Geometry: final body of the model. Coordinates: model frame, mm. Face numbers are marked on the shaded views. A direction names the side the tool comes from. Give positions to 0.01 mm unless a question says otherwise; leave off trailing zeros. Write each loop counter-clockwise with the first axis right and the second up, starting at its lowest first coordinate (ties: lowest second). Pieces come first, ordered by that corner, then holes. Notation, with made-up numbers: M 22.25,-15.75 L 67.25,-15.75 A26 cw 67.25,11.25 Z; hole C 76.25,86 d4. An arc over 180 degrees is marked long. Answer as a JSON object with one key per item and string values.
from build123d import *

# Parameters (mm, degrees)
BASE_FLANGE1_DEPTH = 12.319
FILLET1_RADIUS     = 12.319
FILLET1_LENGTH     = 1.524
FILLET2_RADIUS     = 12.319
FILLET2_LENGTH     = 1.524
SKETCH3_R          = 4.0132
SKETCH3_R_2        = 1.143
EXTRUDE1_DEPTH     = 68.388191377
SKETCH4_R          = 4.0132
SKETCH4_R_2        = 1.143
EXTRUDE2_DEPTH     = 1.524


# Sheet-metal steps are written as plain solids
with BuildPart() as part:
    # Sketch1 → Base-Flange1 (new, symmetric)
    with BuildSketch(Plane.XY):
        with BuildLine():
            Line((-26.162, 40.64), (-26.162, 2.3368))
            ThreePointArc((-26.162, 2.3368), (-25.477567126, 0.684432874), (-23.8252, 0))
            Line((-23.8252, 0), (23.8252, 0))
            ThreePointArc((23.8252, 0), (25.477567126, 0.684432874), (26.162, 2.3368))
            Line((26.162, 2.3368), (26.162, 40.64))
            Line((26.162, 40.64), (24.638, 40.64))
            Line((24.638, 40.64), (24.638, 2.3368))
            ThreePointArc((24.638, 2.3368), (24.399936392, 1.762063608), (23.8252, 1.524))
            Line((23.8252, 1.524), (-23.8252, 1.524))
            ThreePointArc((-23.8252, 1.524), (-24.399936392, 1.762063608), (-24.638, 2.3368))
            Line((-24.638, 2.3368), (-24.638, 40.64))
            Line((-24.638, 40.64), (-26.162, 40.64))
        make_face()
    extrude(amount=BASE_FLANGE1_DEPTH, both=True)

    # Fillet1: full round fillet: the end face becomes a half cylinder, R = half its width
    fillet1_face = Plane((-25.4, 40.64, 0), x_dir=(-1, 0, 0), z_dir=(0, 1, 0))  # on the end face: x along it, z out of the body
    fillet1_slab = fillet1_face.offset(-FILLET1_RADIUS / 2) * Box(FILLET1_LENGTH, 2 * FILLET1_RADIUS, FILLET1_RADIUS, mode=Mode.PRIVATE)  # the body's end, R deep
    fillet1_round = Plane((-25.4, 28.321, 0), x_dir=(0, 1, 0), z_dir=(-1, 0, 0)) * Cylinder(FILLET1_RADIUS, FILLET1_LENGTH, mode=Mode.PRIVATE)  # its axis R under the face
    add(fillet1_slab - fillet1_round, mode=Mode.SUBTRACT)

    # Fillet2: full round fillet: the end face becomes a half cylinder, R = half its width
    fillet2_face = Plane((25.4, 40.64, 0), x_dir=(-1, 0, 0), z_dir=(0, 1, 0))  # on the end face: x along it, z out of the body
    fillet2_slab = fillet2_face.offset(-FILLET2_RADIUS / 2) * Box(FILLET2_LENGTH, 2 * FILLET2_RADIUS, FILLET2_RADIUS, mode=Mode.PRIVATE)  # the body's end, R deep
    fillet2_round = Plane((25.4, 28.321, 0), x_dir=(0, 1, 0), z_dir=(-1, 0, 0)) * Cylinder(FILLET2_RADIUS, FILLET2_LENGTH, mode=Mode.PRIVATE)  # its axis R under the face
    add(fillet2_slab - fillet2_round, mode=Mode.SUBTRACT)

    # Sketch3 → Extrude1 (cut, through all)
    with BuildSketch(Plane(origin=(26.162, 0, 0), x_dir=(0, 0, -1), z_dir=(1, 0, 0))):
        with Locations((0, 28.321)):
            Circle(SKETCH3_R)
        with Locations((0, 36.6522)):
            Circle(SKETCH3_R_2)
        with Locations((8.3312, 28.321)):
            Circle(SKETCH3_R_2)
        with Locations((0, 19.9898)):
            Circle(SKETCH3_R_2)
        with Locations((-8.3312, 28.321)):
            Circle(SKETCH3_R_2)
    extrude(amount=-EXTRUDE1_DEPTH, mode=Mode.SUBTRACT)

    # Sketch4 → Extrude2 (cut)
    with BuildSketch(Plane(origin=(0, 1.524, 0), x_dir=(1, 0, 0), z_dir=(0, 1, 0))):
        with Locations(Location((0, 0, 0), (0, 0, 270))):
            Circle(SKETCH4_R)
        with Locations(Location((0, 8.3312, 0), (0, 0, 270))):
            Circle(SKETCH4_R_2)
        with Locations(Location((8.3312, 0, 0), (0, 0, 270))):
            Circle(SKETCH4_R_2)
        with Locations(Location((0, -8.3312, 0), (0, 0, 270))):
            Circle(SKETCH4_R_2)
        with Locations(Location((-8.3312, 0, 0), (0, 0, 270))):
            Circle(SKETCH4_R_2)
    extrude(amount=-EXTRUDE2_DEPTH, mode=Mode.SUBTRACT)


solid = part.part
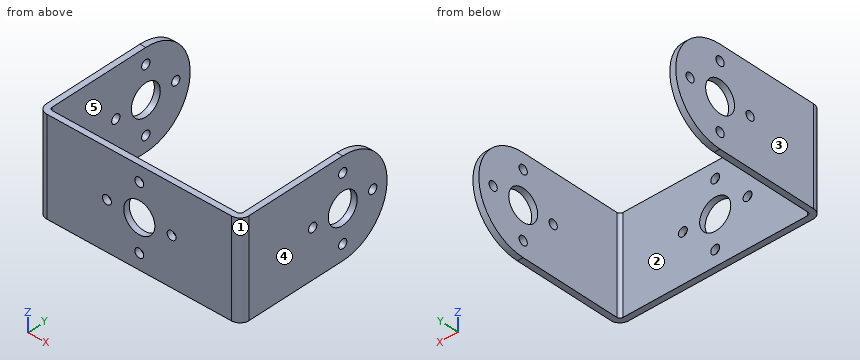
1) Cut plane B-B on y = 11. Return loops of the section in (x, z).
Geometry check:
{"outline": "M -26.16,-12.32 L -24.64,-12.32 L -24.64,12.32 L -26.16,12.32 Z; M 24.64,-12.32 L 26.16,-12.32 L 26.16,12.32 L 24.64,12.32 Z"}
2) Set-up query: the marked faces 4 and 5. Return all of +Z, -Z, +X, -X, +Y, -Y with unobstructed straight access to the full face (end or side cutting, diameter ignored); none if empty.
Geometry check:
{"face 4": "+Z, -Z, +X, +Y, -Y", "face 5": "+Z, -Z, +Y"}
3) Line query: line 1 (X direction, y = 24, z = 10); line 2 (Y direction, x = 25.35, z = 0); line 3 (Y direction, x = -23.5, z = 7.25). Output: solid intervals per line, ascending. Write a range as from..to.
Geometry check:
{"line 1": "x = -26.16..-24.64, 24.64..26.16", "line 2": "y = 0.57..18.85, 21.13..24.31, 32.33..35.51, 37.8..40.64", "line 3": "y = 0..1.52"}
4) Cut plane D-D on y = 31. Return loops of the section in (x, z), and give its area (3 significant figures).
Geometry check:
{"outline": "M -26.16,-12.02 L -24.64,-12.02 L -24.64,-2.99 L -26.16,-2.99 Z; M -26.16,2.99 L -24.64,2.99 L -24.64,12.02 L -26.16,12.02 Z; M 24.64,-12.02 L 26.16,-12.02 L 26.16,-2.99 L 24.64,-2.99 Z; M 24.64,2.99 L 26.16,2.99 L 26.16,12.02 L 24.64,12.02 Z", "area": "55.1 mm2"}
5) Contact query for flat-ended pins moving along their axis: P1, Ø1.8, axis at y = 28.32, z = -8.33, coming from the +X side; P2, Ø1, axis at x = 15, z = -6.5, coming from the -Y side; P3, Ø3, axis at x = -8.33, z = 0, coming from the +Y side. Output: stop coordinate, or through.
Geometry check:
{"P1": "passes through", "P2": "stops at y = 0", "P3": "stops at y = 1.52"}
6) Cut plane A-A on x = 0. Return loops of the section in (y, z), and give its area (3 significant figures).
Geometry check:
{"outline": "M 0,-12.32 L 1.52,-12.32 L 1.52,-9.47 L 0,-9.47 Z; M 0,-7.19 L 1.52,-7.19 L 1.52,-4.01 L 0,-4.01 Z; M 0,4.01 L 1.52,4.01 L 1.52,7.19 L 0,7.19 Z; M 0,9.47 L 1.52,9.47 L 1.52,12.32 L 0,12.32 Z", "area": "18.3 mm2"}
7) Cut plane C-C on z = -1.75. Return loops of the section in (x, y).
Geometry check:
{"outline": "M -26.16,2.34 A2.34 ccw -23.83,0 L -3.61,0 L -3.61,1.52 L -23.83,1.52 A0.81 cw -24.64,2.34 L -24.64,24.71 L -26.16,24.71 Z; M -26.16,31.93 L -24.64,31.93 L -24.64,40.52 L -26.16,40.52 Z; M 3.61,0 L 23.83,0 A2.34 ccw 26.16,2.34 L 26.16,24.71 L 24.64,24.71 L 24.64,2.34 A0.81 cw 23.83,1.52 L 3.61,1.52 Z; M 24.64,31.93 L 26.16,31.93 L 26.16,40.52 L 24.64,40.52 Z"}
8) Pull-direction query (X, two-part tool) for the marked faces 1, 2 and 3; classes: pulls with the +X half, pulls with the -X half, needs draft (parallel to the pull), parting line crosses it, or undercut.
Geometry check:
{"face 1": "pulls with the +X half", "face 2": "undercut", "face 3": "pulls with the -X half"}
